Geometry: final body of the model. Coordinates: model frame, mm. A direction names the side the tool comes from. Give positions to 0.01 mm unless a question says otherwise; leave off trailing zeros. Write each loop counter-clockwise with the first axis right and the second up, starting at its lowest first coordinate (ties: lowest second). Pieces come first, ordered by that corner, then holes.
Q1. Cut plane D-D on y = 3.8. Return the cut outline in (x, z), plus the area to 3 significant figures.
Q2. Cut plane C-C on z = 6. Return the cut outline in (x, y).
Q3. Pin query (flat end, axial travel): pin 1 (2 mm diameter, centred on x = 6, y = 4, fed in from -Z); pin 2 (1.5 mm diameter, centred on x = 4, z = 0, fed in from -Y). Return the tip coordinate at first contact, or that it passes through.
Q4. Cut plane A-A on z = 0. Return the cut outline in (x, y).
Q5. Draft query along X for faces 1 (the face through (5, 1, 6.7)), 2 (the face through (6.91, 3.99, 0.94)), 3 (the face through (1, 0, 0)), 4 (the face through (0.682, 2, 0)). Return one class per face: pulls with the +X half, pulls with the -X half, needs draft (parallel to the pull), parting line crosses it, or undercut.
Q6. Line query: L1, parallel to X at y = 3.8, z = 0; L2, parallel to Z at x = 3.25, y = 1.05; L3, parallel to Y at x = 2, z = 2.5. Output: solid intervals per line, ascending.
Q7. Reachability of faces 5 (the face through (4.7, 4, -2)), 6 (the face through (1.882, 1, 0)), 7 (the face through (5, 2, 7.9)) from +Z, -Z, +X, -X, +Y, -Y: full face, straight path, thin tool, end or side. Return the list, or none.
Q8. Cut plane B-B on x = 5. Return the cut outline in (y, z), plus the area to 3 significant figures.
```python
from build123d import *

# Parameters (mm, degrees)
MAINBASESKETCH_W                 = 7.9
MAINBASESKETCH_H                 = 3.2
MAINBASEEXTRUDE_DEPTH            = 7.9
MAINBASESHELL_T                  = -1.2
SLIMYELLOWUNDEREXT_START         = -0.2
SLIMYELLOWUNDEREXT_DEPTH         = 2
SLIMYELLLOWUPPERCIRCLESKETCH_R   = 2.45
SLIMYELLLOWUPPERCIRCLESKETCH_R_2 = 2
SLIMYELLOWUPPERCIRCLE_DEPTH      = 1.6


with BuildPart() as part:
    # MainBaseSketch → MainBaseExtrude (new, symmetric)
    with BuildSketch(Plane.XY):
        with Locations((4.631967213, 1.6)):
            Rectangle(MAINBASESKETCH_W, MAINBASESKETCH_H)
    extrude(amount=MAINBASEEXTRUDE_DEPTH, both=True)

    # MainBaseShell
    mainbaseshell_openings = [part.faces().sort_by_distance(p)[0] for p in [
        (4.631967213, 0, 0),
    ]]
    offset(amount=MAINBASESHELL_T, openings=mainbaseshell_openings, kind=Kind.INTERSECTION)

    # SlimYellowUnderExtSketch → SlimYellowUnderExt (add)
    with BuildSketch(Plane.XZ.offset(-2).offset(SLIMYELLOWUNDEREXT_START)):
        Polygon((6.683445552, 2.45), (7.181967213, 2.947188682), (7.381967213, 2.947188682), (7.381967213, 1.952811318), (7.181967213, 1.952811318), align=None)
        Polygon((1.881967213, 1.952811318), (1.881967213, 2.947188682), (2.081967213, 2.947188682), (2.580488874, 2.45), (2.081967213, 1.952811318), align=None)
        Polygon((2.580488874, -2.45), (2.081967213, -2.947188682), (1.881967213, -2.947188682), (1.881967213, -1.952811318), (2.081967213, -1.952811318), align=None)
        Polygon((6.683445552, -2.45), (7.181967213, -1.952811318), (7.381967213, -1.952811318), (7.381967213, -2.947188682), (7.181967213, -2.947188682), align=None)
    extrude(amount=SLIMYELLOWUNDEREXT_DEPTH)

    # SlimYelllowUpperCircleSketch → SlimYellowUpperCircle (add)
    with BuildSketch(Plane(origin=(0, 3.2, 0), x_dir=(1, 0, 0), z_dir=(0, 1, 0))):
        with Locations((4.647335619, 0)):
            Circle(SLIMYELLLOWUPPERCIRCLESKETCH_R)
        with Locations(Location((4.647335619, 0, 0), (0, 0, 270))):
            Circle(SLIMYELLLOWUPPERCIRCLESKETCH_R_2, mode=Mode.SUBTRACT)
    extrude(amount=SLIMYELLOWUPPERCIRCLE_DEPTH)


solid = part.part
```
Data:
1. outline: circle Ø4.9 at (4.65, 0); hole circle Ø4 at (4.65, 0)
1. area: 6.29 mm2
2. outline: (0.68, 0) - (1.88, 0) - (1.88, 2) - (7.38, 2) - (7.38, 0) - (8.58, 0) - (8.58, 3.2) - (0.68, 3.2) - close
3. pin 1: stops at z = -7.9
3. pin 2: stops at y = 2
4. outline: (0.68, 0) - (1.88, 0) - (1.88, 2) - (7.38, 2) - (7.38, 0) - (8.58, 0) - (8.58, 3.2) - (7.1, 3.2) - (7.1, 4.8) - (6.65, 4.8) - (6.65, 3.2) - (2.65, 3.2) - (2.65, 4.8) - (2.2, 4.8) - (2.2, 3.2) - (0.68, 3.2) - close
5. face 1: undercut
5. face 2: parting line crosses it
5. face 3: needs draft
5. face 4: pulls with the -X half
6. L1: x = 2.2 to 2.65, 6.65 to 7.1
6. L2: z = -7.9 to -6.7, 6.7 to 7.9
6. L3: y = 0.2 to 3.2
7. face 5: +Y
7. face 6: -Y
7. face 7: +Z, +X, -X, +Y, -Y
8. outline: (0, -7.9) - (3.2, -7.9) - (3.2, -2.42) - (4.8, -2.42) - (4.8, -1.97) - (3.2, -1.97) - (3.2, 1.97) - (4.8, 1.97) - (4.8, 2.42) - (3.2, 2.42) - (3.2, 7.9) - (0, 7.9) - (0, 6.7) - (2, 6.7) - (2, -6.7) - (0, -6.7) - close
8. area: 25.2 mm2
